Solid Edge part; units mm, degrees
sketch "Sketch1" plane through (0, 0, 0) normal (0, -1, 0) x (1, 0, 0)
  line L0 (9.525, 12.7) -> (-9.525, 12.7)
  arc A0 (-9.525, 12.7) -> (-12.7, 9.525) centre (-9.525, 9.525) ccw
  line L1 (-12.7, 9.525) -> (-12.7, -9.525)
  arc A1 (-9.525, -12.7) -> (-12.7, -9.525) centre (-9.525, -9.525) cw
  line L2 (-9.525, -12.7) -> (9.525, -12.7)
  arc A2 (9.525, -12.7) -> (12.7, -9.525) centre (9.525, -9.525) ccw
  line L3 (12.7, -9.525) -> (12.7, 9.525)
  arc A3 (12.7, 9.525) -> (9.525, 12.7) centre (9.525, 9.525) ccw
  line L4 (9.525, 11.176) -> (-9.525, 11.176)
  arc A4 (-9.525, 11.176) -> (-11.176, 9.525) centre (-9.525, 9.525) ccw
  line L5 (-11.176, 9.525) -> (-11.176, -9.525)
  arc A5 (-11.176, -9.525) -> (-9.525, -11.176) centre (-9.525, -9.525) ccw
  line L6 (-9.525, -11.176) -> (9.525, -11.176)
  arc A6 (9.525, -11.176) -> (11.176, -9.525) centre (9.525, -9.525) ccw
  line L7 (11.176, -9.525) -> (11.176, 9.525)
  arc A7 (11.176, 9.525) -> (9.525, 11.176) centre (9.525, 9.525) ccw
extrude "Protrusion1" add sketch "Sketch1" along normal mid plane 25.4
properties material "Steel"
CAD build for the part. Positions are in the model's coordinates, mm. A direction names the side the tool comes from. Round coordinates to 2 decimals unless told otherwise and drop trailing zeros. Write each loop counter-clockwise with the first axis right and the second up, starting at its lowest first coordinate (ties: lowest second). Pieces come first, ordered by that corner, then holes. Notation, with made-up numbers: (-33, -19) -> (-6, -19) arc R17 cw to (-6, 7) -> close; hole circle Ø11 at (72.5, 54). An arc over 180 degrees is marked (long way). Answer in a Markdown table with one row per item. Add a question column.
Item 1: Saw through at C-C, the plane z = -8. Write the cut outline in (x, y), then the cut area to 3 significant figures.
Item 2: Saw through at A-A, the plane x = 1. Write the cut outline in (y, z).
Item 3: Which spindle directions (+Z, -Z, +X, -X, +Y, -Y) get a long thin tool onto all of the face, cutting with end or side? Do faces 4 (the face through (12.7, 0, 0)), 5 (the face through (-11.176, 0, 0)). Say none if no direction does.
Item 4: Mould opens along Z. For faces 1 (the face through (10.705, 0.178, -10.68)), 2 (the face through (-11.79, 0.18, 11.75)), 3 (the face through (1, 12.7, 11.35)) say: pulls with the +Z half, pulls with the -Z half, needs draft (parallel to the pull), parting line crosses it, or undercut.
Item 5: Drill centre lines: line 1 (X direction, y = 10.5, z = -0.75); line 2 (X direction, y = 11.75, z = -10.75). Where is each one in solid material? Low to high. Write a range as from..to.
Item 6: Drop a flat-ended pin along its axis: pin 1 Ø6 at (x, z) = (-6, -3) entering from -Y. Give the stop position or say it passes through.
Item 7: Saw through at B-B, the plane y = 2.25. Write the cut outline in (x, z) (3 decimals), then the cut area to 3 significant figures.
Findings below:
| question | item | result |
|---|---|---|
| 1 | outline | (-12.7, -12.7) -> (-11.18, -12.7) -> (-11.18, 12.7) -> (-12.7, 12.7) -> close; (11.18, -12.7) -> (12.7, -12.7) -> (12.7, 12.7) -> (11.18, 12.7) -> close |
| 1 | area | 77.4 mm^2 |
| 2 | outline | (-12.7, -12.7) -> (12.7, -12.7) -> (12.7, -11.18) -> (-12.7, -11.18) -> close; (-12.7, 11.18) -> (12.7, 11.18) -> (12.7, 12.7) -> (-12.7, 12.7) -> close |
| 3 | face 4 | +Z, -Z, +X, +Y, -Y |
| 3 | face 5 | +Y, -Y |
| 4 | face 1 | undercut |
| 4 | face 2 | pulls with the +Z half |
| 4 | face 3 | needs draft |
| 5 | line 1 | x = -12.7..-11.18, 11.18..12.7 |
| 5 | line 2 | x = -12.45..-10.63, 10.63..12.45 |
| 6 | pin 1 | passes through |
| 7 | outline | (-12.7, -9.525) arc R3.175 ccw to (-9.525, -12.7) -> (9.525, -12.7) arc R3.175 ccw to (12.7, -9.525) -> (12.7, 9.525) arc R3.175 ccw to (9.525, 12.7) -> (-9.525, 12.7) arc R3.175 ccw to (-12.7, 9.525) -> close; hole (-11.176, -9.525) arc R1.651 ccw to (-9.525, -11.176) -> (9.525, -11.176) arc R1.651 ccw to (11.176, -9.525) -> (11.176, 9.525) arc R1.651 ccw to (9.525, 11.176) -> (-9.525, 11.176) arc R1.651 ccw to (-11.176, 9.525) -> close |
| 7 | area | 139 mm^2 |
